Part print with two shaded views. Sizes in mm from the minimum x, y, z corner. A direction names the side the tool comes from. Give positions to 0.01 mm unless a question says otherwise; leave off trailing zeros. Write each loop counter-clockwise with the first axis right and the second up, starting at its lowest first coordinate (ties: lowest second). Pieces come first, ordered by that corner, then holes. Notation, with made-up numbers: M 35,-40 L 46,-40 A22 ccw 46,-10 Z; hole C -39,40.5 d10. An arc over 180 degrees is marked long. Return JSON: item names as keys, results as strings. Group by question number.
Q1. Wall check: probe 1 along Y at (x, z) = (6, 3.5); probe 2 along X at (y, z) = (6, 7); probe 3 along X at (y, z) = (10.5, 7.6). Give the ranges that are in metal, low to high.
Q2. Band-saw the part on B-B, the plane x = 22. Give the cut face in (y, z), then the cut area to 3 significant figures.
Q3. Tool access for the marked faces 4, 5, 6 and 7: list every direction of +Z, -Z, +X, -X, +Y, -Y with a clear straight run to the whole face (end or side of a thin tool).
Q4. Band-saw the part on D-D, the plane x = 29. Give the cut face in (y, z).
Q5. Band-saw the part on C-C, the plane z = 6.75. Count the separate pieces of the cut face and the enclosed holes in it, then the cut area to 3 significant figures.
Q6. Flat gauge pins, fed straight in: pin 1 Ø16.5 at (x, y) = (39, 17.5) entering from +Z; pin 2 Ø6 at (x, z) = (22, 7.6) entering from +Y; pin 3 Ø5 at (x, y) = (25, 16.5) entering from -Z. Where does each tip first touch, or does it go through?
Q7. Pull direction Y, two halves, no side cores. Call the marked faces 1, 2 and 3: +Y half, -Y half, draft (parallel to the pull), parting line (faces both ways), or undercut.
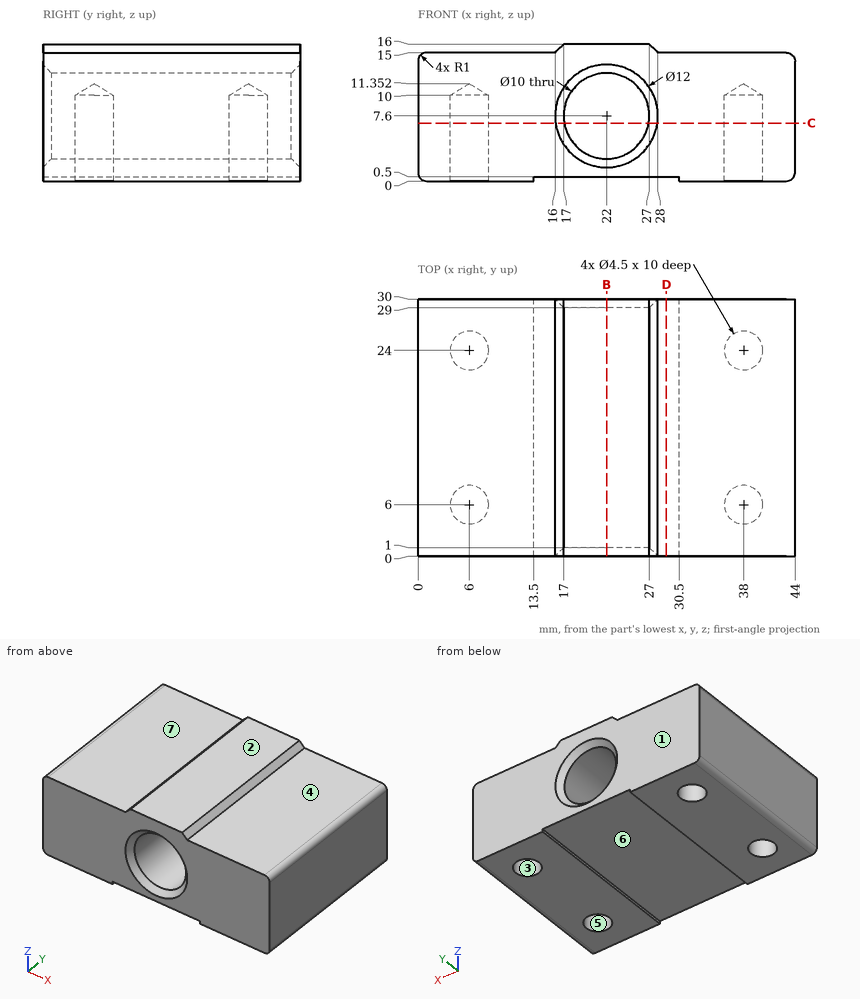
From the geometry:
{
 "1": {"probe 1": "y = 0 to 3.75, 8.25 to 21.75, 26.25 to 30", "probe 2": "x = 0 to 3.75, 8.25 to 17.04, 26.96 to 35.75, 40.25 to 44", "probe 3": "x = 0 to 17, 27 to 44"},
 "2": {"outline": "M 0,0.5 L 30,0.5 L 30,1.6 L 29,2.6 L 1,2.6 L 0,1.6 Z; M 0,13.6 L 1,12.6 L 29,12.6 L 30,13.6 L 30,16 L 0,16 Z", "area": "163 mm^2"},
 "3": {"face 4": "+Z, +X, +Y, -Y", "face 5": "-Z", "face 6": "-Z, +Y, -Y", "face 7": "+Z, -X, +Y, -Y"},
 "4": {"outline": "M 0,0.5 L 30,0.5 L 30,15 L 0,15 Z"},
 "5": {"separate pieces": "2", "enclosed holes": "4", "area": "959 mm^2"},
 "6": {"pin 1": "stops at z = 15", "pin 2": "passes through", "pin 3": "stops at z = 0.5"},
 "7": {"face 1": "+Y half", "face 2": "draft", "face 3": "undercut"}
}
